Can you work these out from the model? Positions are in its coordinate system, mm. A direction names the side the tool comes from. Give positions to 0.01 mm unless a question says otherwise; leave off trailing zeros. Order: outer loops, then holes, each group sorted by start corner. A loop starts at its lowest first (then second) coordinate and runs counter-clockwise, first axis right, second up. Notation, with made-up numbers: M -22.75,-25.5 L 2.25,-25.5 A11 cw 2.25,-19.5 Z; hole C -31.75,32 d7. An arc over 180 degrees is marked long. One line per question, with ' | ' between items. Start each with the question number.
1) If we section it at C-C, the plane x = 22.5: Please give me the cut outline in (y, z).
2) If we section it at B-B, the plane y = 26.5: Please give me the cut outline in (x, z), plus the area to 3 significant figures.
3) Thinking about a two-plate mould opening in Z: for faces 1 (the flat face through (-12, 17, 33.93)), 2 (the flat face through (6, -3, 23)), 3 (the cylindrical face through (42.309, -1.479, 25.568)), which applies, +Z half, -Z half, draft (parallel to the pull), parting line (faces both ways), or undercut?
4) For faces 4 (the flat face through (-22, 0, 25.501)), 5 (the flat face through (30.538, 6.5, 16)), 6 (the flat face through (36, 0, 27.03)), 7 (the cylindrical face through (30.93, 3.46, 26.51)), which set-ups out of +Z, -Z, +X, -X, +Y, -Y let a thin tool reach every point of the face, with its end or its side?
5) I'm going to push flat-ended pins straight in: pin 1 Ø1.5 at (y, z) = (13, 18) entering from +X; pin 2 Ø3.5 at (x, y) = (-10.36, 26.5) entering from -Z; pin 3 Ø1.3 at (x, y) = (31, 21.5) entering from +Z; pin 4 Ø5 at (x, z) = (-25.36, 20.5) entering from +Y. Where does each tip first touch, or does it pass through?
6) Please list where these lines run through material, in increasing order: line 1 along Z through (x, y) = (10, 17); line 2 along Y through (x, z) = (-11, 11.25); line 3 along X through (y, z) = (28.5, 11). Write a range as [from, to].
7) If we section it at D-D, the plane z = 11: Please give me the cut outline in (x, y).
8) If we section it at A-A, the plane y = 18.5: Please give me the cut outline in (x, z), plus the area to 3 significant figures.
Autodesk Inventor part; units mm, degrees
ref_plane "YZ Plane" through (0, 0, 0) normal (1, 0, 0) x (0, 1, 0)
ref_plane "XZ Plane" through (0, 0, 0) normal (0, 1, 0) x (-1, 0, 0)
ref_plane "XY Plane" through (0, 0, 0) normal (0, 0, 1) x (1, 0, 0)
sketch "Sketch1" plane through (0, 0, 0) normal (0, 1, 0) x (-1, 0, 0)
  line L0 (17.1623, 10.1297) -> (-30.5377, 10.1297)
  line L1 (-30.5377, 34.9297) -> (7.4623, 34.9297)
  line L2 (7.4623, 34.9297) -> (7.4623, 33.9297)
  line L3 (7.4623, 33.9297) -> (17.1623, 33.9297)
  line L4 (17.1623, 33.9297) -> (17.1623, 10.1297)
  line L5 (-31.7377, 8.9297) -> (18.3623, 8.9297)
  line L6 (18.3623, 8.9297) -> (18.3623, 35.1297)
  line L7 (18.3623, 35.1297) -> (8.6623, 35.1297)
  line L8 (8.6623, 35.1297) -> (8.6623, 36.1297)
  line L9 (8.6623, 36.1297) -> (-31.7377, 36.1297)
  line L10 (-30.5377, 10.1297) -> (-30.5377, 34.9297)
  line L11 (-31.7377, 8.9297) -> (-31.7377, 36.1297)
  point P0 (0, 0)
  dimension "d0" = 47.7
  dimension "d1" = 23.8
  dimension "d2" = 9.7
  dimension "d3" = 1
  dimension "d4" = 1.2
  dimension "d5" = 1.2
  dimension "d6" = 1.2
  dimension "d7" = 1.2
  dimension "d8" = 1.2
  dimension "d19" = 1.2
extrude "Extrusion3" add sketch "Sketch1" along normal blind 33.5
sketch "Sketch3" plane through (0, 0, 0) normal (0, -1, 0) x (1, 0, 0)
  line L0 (30.5377, 34.9297) -> (-7.4623, 34.9297)
  line L1 (30.5377, 34.9297) -> (30.5377, 10.1297)
  line L2 (30.5377, 34.9297) -> (30.5377, 10.1297)
  line L3 (-17.1623, 10.1297) -> (30.5377, 10.1297)
  line L4 (30.5377, 10.1297) -> (-17.1623, 10.1297)
  line L5 (-17.1623, 33.9297) -> (-17.1623, 10.1297)
  line L6 (-17.1623, 10.1297) -> (-17.1623, 33.9297)
  line L7 (-7.4623, 33.9297) -> (-7.4623, 34.9297)
  line L8 (-17.1623, 33.9297) -> (-7.4623, 33.9297)
  line L9 (-7.4623, 33.9297) -> (-7.4623, 34.9297)
  line L10 (-7.4623, 34.9297) -> (30.5377, 34.9297)
  point P0 (0, 0)
extrude "Extrusion4" add sketch "Sketch3" against normal blind 1.2
sketch "Sketch4" plane through (31.7377, 0, 8.9297) normal (0, 0, -1) x (-1, 0, 0)
  arc A0 (29.9, 16.8) -> (38.3, 16.8) centre (34.1, 16.8) ccw
  line L0 (50.1, 0) -> (50.1, 33.5)
  line L1 (0, 0) -> (50.1, 0)
  line L2 (29.9, 16.8) -> (29.9, 33.5)
  line L3 (29.9, 33.5) -> (38.3, 33.5)
  line L4 (0, 33.5) -> (50.1, 33.5)
  line L5 (38.3, 33.5) -> (38.3, 16.8)
  circle A1 centre (42.1, 26.5) radius 2
  circle A2 centre (42.1, 8.5) radius 2
  circle A3 centre (9.1, 8.5) radius 2
  circle A4 centre (9.1, 26.5) radius 2
  line L6 (0, 0) -> (0, 33.5)
  point P0 (31.7377, 0)
  dimension "d24" = 16
  dimension "d25" = 16.8
  dimension "d26" = 4.2
  dimension "d27" = 4
  dimension "d29" = 7
  dimension "d30" = 4
  dimension "d32" = 18
  dimension "d33" = 4
  dimension "d34" = 4
  dimension "d36" = 18
  dimension "d37" = 7
  dimension "d38" = 0
  dimension "d63" = 33
  dimension "d64" = 8
extrude "Extrusion5" cut sketch "Sketch4" against normal blind 5 contours L2 L3 L5 A0 | A1 | A2 | A3 | A4
sketch "Sketch5" plane through (31.7377, 0, 36.1297) normal (1, 0, 0) x (0, 0, -1)
  arc A0 (-0.7, 15.6) -> (23.9, 15.6) centre (11.6, 15.6) ccw
  line L0 (0, 0) -> (27.2, 0)
  line L1 (27.2, 0) -> (27.2, 33.5)
  line L2 (23.9, 15.6) -> (23.9, 33.5)
  line L3 (27.2, 33.5) -> (1, 33.5)
  line L4 (1, 33.5) -> (0, 33.5)
  line L5 (-0.7, 15.6) -> (18, 15.6) construction
  line L6 (0.1, 33.5) -> (23.9, 33.5)
  line L7 (-0.7, 15.6) -> (0, 15.6)
  line L8 (0, 0) -> (0, 33.5)
  line L9 (0, 15.6) -> (0, 33.5)
  line L10 (0, 33.5) -> (0.1, 33.5)
  point P0 (36.1297, 0)
  dimension "d41" = 24.6
  dimension "d42" = 15.6
  dimension "d43" = 15.6
extrude "Extrusion6" cut sketch "Sketch5" against normal blind 3 contours L7 L8 A0 | L8 L4 L3 L2 A0
sketch "Sketch6" plane through (0, 0, 0) normal (0, -1, 0) x (1, 0, 0)
  line L0 (39.3039, 27.0297) -> (31.7377, 27.0297)
  line L1 (31.7377, 27.0297) -> (31.7377, 17.0297)
  line L2 (31.7377, 17.0297) -> (38.7377, 17.0297)
  line L3 (43.7377, 21.6451) -> (43.7377, 22.4464)
  line L4 (31.7377, 36.1297) -> (31.7377, 8.9297)
  line L5 (31.7377, 8.9297) -> (-18.3623, 8.9297)
  arc A0 (38.7377, 17.0297) -> (39.3039, 27.0297) centre (38.7377, 22.0458) ccw
  line L6 (-18.3623, 8.9297) -> (-18.3623, 35.1297)
  line L7 (-18.3623, 25.5012) -> (-25.3623, 25.5012)
  line L8 (-30.3623, 15.5012) -> (-18.3623, 15.5012)
  line L9 (-18.3623, 15.5012) -> (-18.3623, 25.5012)
  arc A1 (-25.3623, 25.5012) -> (-25.3623, 15.5012) centre (-25.3623, 20.5012) ccw
  circle A2 centre (-25.3623, 20.5012) radius 3
  circle A3 centre (38.7377, 22.0458) radius 3
  point P0 (0, 0)
  dimension "d48" = 10
  dimension "d49" = 0
  dimension "d50" = 8.1
  dimension "d51" = 5
  dimension "d52" = 7
  dimension "d53" = 12
  dimension "d55" = 7
  dimension "d56" = 6
  dimension "d57" = 6
extrude "Extrusion7" add sketch "Sketch6" against normal blind 3.3 contours A0 L3 L2 L1 L0 | L8 A1 L7 L6
sketch "Sketch7" plane through (0, 0, 0) normal (0, -1, 0) x (1, 0, 0)
  circle A0 centre (-25.3623, 20.5012) radius 3
  circle A1 centre (38.7377, 22.0458) radius 3
  line L0 (31.7377, 8.9297) -> (-18.3623, 8.9297)
  line L1 (31.7377, 17.0297) -> (31.7377, 8.9297)
  line L2 (31.7377, 17.0297) -> (38.7377, 17.0297)
  arc A2 (38.7377, 17.0297) -> (43.7377, 21.6451) centre (38.7377, 22.0458) ccw
  line L3 (43.7377, 21.6451) -> (43.7377, 22.4464)
  arc A3 (43.7377, 22.4464) -> (39.3039, 27.0297) centre (38.7377, 22.0458) ccw
  line L4 (39.3039, 27.0297) -> (31.7377, 27.0297)
  line L5 (31.7377, 36.1297) -> (31.7377, 27.0297)
  line L6 (-8.6623, 36.1297) -> (31.7377, 36.1297)
  line L7 (-8.6623, 35.1297) -> (-8.6623, 36.1297)
  line L8 (-18.3623, 35.1297) -> (-8.6623, 35.1297)
  line L9 (-18.3623, 25.5012) -> (-18.3623, 35.1297)
  line L10 (-18.3623, 25.5012) -> (-25.3623, 25.5012)
  arc A4 (-25.3623, 25.5012) -> (-25.3623, 15.5012) centre (-25.3623, 20.5012) ccw
  line L11 (-25.3623, 15.5012) -> (-18.3623, 15.5012)
  line L12 (-18.3623, 8.9297) -> (-18.3623, 15.5012)
  point P0 (0, 0)
extrude "Extrusion8" add sketch "Sketch7" along normal blind 3
properties part number "MotorMount"
Results found:
1) outline: M -3,8.93 L 6.5,8.93 L 6.5,10.13 L 1.2,10.13 L 1.2,34.93 L 33.5,34.93 L 33.5,36.13 L -3,36.13 Z; M 10.5,8.93 L 24.5,8.93 L 24.5,10.13 L 10.5,10.13 Z; M 28.5,8.93 L 33.5,8.93 L 33.5,10.13 L 28.5,10.13 Z
2) outline: M -18.36,8.93 L -12.36,8.93 L -12.36,10.13 L -17.16,10.13 L -17.16,33.93 L -7.46,33.93 L -7.46,34.93 L 28.74,34.93 L 28.74,36.13 L -8.66,36.13 L -8.66,35.13 L -18.36,35.13 Z; M -8.36,8.93 L -6.56,8.93 L -6.56,10.13 L -8.36,10.13 Z; M 1.84,8.93 L 20.64,8.93 L 20.64,10.13 L 1.84,10.13 Z; M 24.64,8.93 L 31.74,8.93 L 31.74,12.23 L 30.54,12.23 L 30.54,10.13 L 24.64,10.13 Z | area: 129 mm²
3) face 1: undercut | face 2: draft | face 3: +Z half
4) face 4: +Z, -X, +Y, -Y | face 5: +Y | face 6: +Z, +X, +Y, -Y | face 7: +X, +Y
5) pin 1: stops at x = -17.16 | pin 2: stops at z = 33.93 | pin 3: stops at z = 12.23 | pin 4: passes through
6) line 1: z = [8.93, 10.13], [34.93, 36.13] | line 2: y = [-3, 1.2] | line 3: x = [-18.36, -17.16], [30.54, 31.74]
7) outline: M -18.36,-3 L 31.74,-3 L 31.74,33.5 L 30.54,33.5 L 30.54,1.2 L -17.16,1.2 L -17.16,33.5 L -18.36,33.5 Z
8) outline: M -18.36,8.93 L -6.56,8.93 L -6.56,10.13 L -17.16,10.13 L -17.16,33.93 L -7.46,33.93 L -7.46,34.93 L 28.74,34.93 L 28.74,36.13 L -8.66,36.13 L -8.66,35.13 L -18.36,35.13 Z; M 1.84,8.93 L 31.74,8.93 L 31.74,12.23 L 30.54,12.23 L 30.54,10.13 L 1.84,10.13 Z | area: 139 mm²
